```python
from build123d import *

# Parameters (mm, degrees)
SKETCH1_R           = 2.9
BOSS_EXTRUDE1_DEPTH = 13
BOSS_EXTRUDE2_DEPTH = 10
SKETCH3_R           = 1.6
CUT_EXTRUDE1_DEPTH  = 25
CUT_EXTRUDE2_DEPTH  = 7


with BuildPart() as part:
    # Sketch1 → Boss-Extrude1 (new body)
    with BuildSketch(Plane(origin=(0, 0, 0), x_dir=(1, 0, 0), z_dir=(0, 1, 0))):
        with Locations(Location((0, 0, 0), (0, 0, 270))):
            Circle(SKETCH1_R)
    extrude(amount=BOSS_EXTRUDE1_DEPTH)

    # Sketch2 → Boss-Extrude2 (add)
    with BuildSketch(Plane(origin=(0, 13, 0), x_dir=(1, 0, 0), z_dir=(0, 1, 0))):
        Polygon((6.5, 0), (3.25, 5.629165125), (-3.25, 5.629165125), (-6.5, 0), (-3.25, -5.629165125), (3.25, -5.629165125), align=None)
    extrude(amount=BOSS_EXTRUDE2_DEPTH)

    # Sketch3 → Cut-Extrude1 (cut)
    with BuildSketch(Plane.XZ):
        with Locations(Location((0, 0, 0), (0, 0, 270))):
            Circle(SKETCH3_R)
    extrude(amount=-CUT_EXTRUDE1_DEPTH, mode=Mode.SUBTRACT)

    # Sketch4 → Cut-Extrude2 (cut)
    with BuildSketch(Plane(origin=(0, 23, 0), x_dir=(1, 0, 0), z_dir=(0, 1, 0))):
        Polygon((0, 3.2), (-2.771281292, 1.6), (-2.771281292, -1.6), (0, -3.2), (2.771281292, -1.6), (2.771281292, 1.6), align=None)
    extrude(amount=-CUT_EXTRUDE2_DEPTH, mode=Mode.SUBTRACT)


solid = part.part
```
The listing builds one solid part. Answer for the finished solid, in the listing's coordinates (mm). A direction names the side the tool comes from. Coordinates: 2 decimals unless noted, no trailing zeros. Loops run counter-clockwise (first coordinate to the right, second up) from the corner with the lowest first, then second, coordinate; pieces in that order, holes last. Notation, with made-up numbers: (36.25, 51.25) -> (89.25, 51.25) arc R23 ccw to (89.25, 61.25) -> close; hole circle Ø9 at (81.5, 51.5). An arc over 180 degrees is marked (long way). Use one line per item in the form item = value. Start each with the question number.
Item 1: The part is cut by section A-A on y = 17. Determine the outline of the cut face in (x, z).
Item 2: The mould has two halves that part along Z. Classify faces 1 (the face through (-4.898, 17.93, 2.775)), 2 (the face through (1.37, 19.55, 2.41)), 3 (the face through (4.898, 17.93, -2.775)): released by +Z, released by -Z, zero draft, split by the parting line, or undercut.
Item 3: Flat-ended cylindrical pins translate along their axes: pin 1 Ø6 at (x, z) = (-1, 0.5) entering from +Y; pin 2 Ø2 at (x, z) = (3.5, -3) entering from -Y; pin 3 Ø6 at (y, z) = (18.5, 0.5) entering from -X. Find the tip coordinate at first contact, or state that the pin passes through.
Item 4: Consider L1, parallel to X at y = 7, z = 0; L2, parallel to Y at x = 1.75, z = 0; L3, parallel to Y at x = 1.75, z = -3.75. Determine where each line is inside the solid, lowest interval first. Write a range as [from, to].
Item 5: A tool of negligible diameter and unlimited length cuts with its end or side. For faces 4 (the face through (3, 23, 0)), 5 (the face through (-1.37, 19.55, -2.41)), 6 (the face through (0.1, 6.4, -2.9)), from which of +Z, -Z, +X, -X, +Y, -Y can it reach the whole face along a straight path? Write none if from no direction.
Item 6: The part is cut by section B-B on y = 14.25. Determine the outline of the cut face in (x, z).
Item 7: The part is cut by section C-C on z = 2. Determine the outline of the cut face in (x, y), then the cut area to 3 significant figures.
Item 8: The part is cut by section D-D on z = -1.25. Determine the outline of the cut face in (x, y).
Answer key:
q1.outline = (-6.5, 0) -> (-3.25, -5.63) -> (3.25, -5.63) -> (6.5, 0) -> (3.25, 5.63) -> (-3.25, 5.63) -> close; hole (-2.77, -1.6) -> (0, -3.2) -> (2.77, -1.6) -> (2.77, 1.6) -> (0, 3.2) -> (-2.77, 1.6) -> close
q2.face_1 = released by +Z
q2.face_2 = undercut
q2.face_3 = released by -Z
q3.pin_1 = 23
q3.pin_2 = 13
q3.pin_3 = -6.5
q4.L1 = [-2.9, -1.6], [1.6, 2.9]
q4.L2 = [0, 16]
q4.L3 = [13, 23]
q5.face_4 = +Z, -Z, +X, -X, +Y
q5.face_5 = +Y
q5.face_6 = -Y
q6.outline = (-6.5, 0) -> (-3.25, -5.63) -> (3.25, -5.63) -> (6.5, 0) -> (3.25, 5.63) -> (-3.25, 5.63) -> close; hole circle Ø3.2 at (0, 0)
q7.outline = (-5.35, 13) -> (-2.1, 13) -> (-2.1, 0) -> (2.1, 0) -> (2.1, 13) -> (5.35, 13) -> (5.35, 23) -> (2.08, 23) -> (2.08, 16) -> (-2.08, 16) -> (-2.08, 23) -> (-5.35, 23) -> close
q7.area = 132 mm2
q8.outline = (-5.78, 13) -> (-2.62, 13) -> (-2.62, 0) -> (-1, 0) -> (-1, 16) -> (-2.77, 16) -> (-2.77, 23) -> (-5.78, 23) -> close; (1, 0) -> (2.62, 0) -> (2.62, 13) -> (5.78, 13) -> (5.78, 23) -> (2.77, 23) -> (2.77, 16) -> (1, 16) -> close
